```python
from build123d import *

# Parameters (mm, degrees)
SKETCH_1_R          = 1.6
EXTRUDE_1_DEPTH     = 13
SKETCH_2_W          = 16.5
SKETCH_2_H          = 11
CUT_EXTRUDE_1_DEPTH = 41.749969325
SKETCH_3_R          = 1.6
CUT_EXTRUDE_2_DEPTH = 34.189757456
FILLET_2_R          = 5
FILLET_3_R          = 3


with BuildPart() as part:
    # 草图1 → 凸台-拉伸1 (new, symmetric)
    with BuildSketch(Plane.XY):
        Polygon((-10.1, 0), (-10.1, 10), (10.1, 10), (10.1, 0), (13.1, 0), (26.6, 0), (26.6, 28), (10.6, 28), (10.6, 13), (-13.1, 13), (-13.1, 0), align=None)
        with Locations(Location((23.6, 25, 0), (0, 0, 180))):
            Circle(SKETCH_1_R, mode=Mode.SUBTRACT)
        with Locations(Location((13.6, 3, 0), (0, 0, 180))):
            Circle(SKETCH_1_R, mode=Mode.SUBTRACT)
    extrude(amount=EXTRUDE_1_DEPTH, both=True)

    # 草图2 → 切除-拉伸1 (cut, through all)
    with BuildSketch(Plane.XZ):
        with Locations((18.35, 0)):
            Rectangle(SKETCH_2_W, SKETCH_2_H)
    extrude(amount=-CUT_EXTRUDE_1_DEPTH, mode=Mode.SUBTRACT)

    # 草图3 → 切除-拉伸2 (cut, through all)
    with BuildSketch(Plane(origin=(0, 13, 0), x_dir=(1, 0, 0), z_dir=(0, 1, 0))):
        with Locations(Location((0, 10, 0), (0, 0, 180))):
            Circle(SKETCH_3_R)
        with Locations(Location((0, -10, 0), (0, 0, 180))):
            Circle(SKETCH_3_R)
    extrude(amount=-CUT_EXTRUDE_2_DEPTH, mode=Mode.SUBTRACT)

    # 圆角2
    fillet_2_edges = [part.edges().sort_by_distance(p)[0] for p in [
        (10.6, 13, -9.25),
    ]]
    fillet(fillet_2_edges, radius=FILLET_2_R)

    # 圆角3
    fillet_3_edges = [part.edges().sort_by_distance(p)[0] for p in [
        (10.6, 28, 9.25),
        (26.6, 28, 9.25),
        (26.6, 0, 9.25),
        (10.1, 0, 9.25),
        (10.6, 28, -9.25),
        (26.6, 28, -9.25),
        (26.6, 0, -9.25),
        (10.1, 0, -9.25),
    ]]
    fillet(fillet_3_edges, radius=FILLET_3_R)


solid = part.part
```
Build history of the part. All positions in model axes, mm. A direction names the side the tool comes from. Round coordinates to 2 decimals unless told otherwise and drop trailing zeros. Loops run counter-clockwise (first coordinate to the right, second up) from the corner with the lowest first, then second, coordinate; pieces in that order, holes last.
Item 1: Saw through at C-C (y = 10.75). List the corners of the cut face in (x, z), then the cut area to 3 significant figures.
Item 2: Pin check, flat tips, straight feed: P1, Ø3.5, axis at y = 22, z = -8.5, coming from the -X side; P2, Ø5, axis at x = 8.5, z = -10, coming from the +Y side; P3, Ø4, axis at x = 0, z = 10, coming from the +Y side. Stop position of each tip, or through.
Item 3: Drill centre lines: line 1 along X through (y, z) = (3, 8.5); line 2 along Y through (x, z) = (13.5, 11.5); line 3 along Y through (x, z) = (23.6, 7.5). Where is each one in solid material? Low to high.
Item 4: Saw through at A-A (z = -10). List the corners of the cut face in (x, y).
Item 5: Saw through at B-B (x = 0). List the corners of the cut face in (y, z), then the cut area to 3 significant figures.
Item 6: Saw through at D-D (x = 17). List the corners of the cut face in (y, z).
Item 7: Which spindle directions (+Z, -Z, +X, -X, +Y, -Y) get a long thin tool onto all of the face, cutting with end or side? Do faces 5 (the face through (10.6, 22, 9)), 6 (the face through (25.7, 27.14, -9.2)), 7 (the face through (0, 10, 0)). Say none if no direction does.
Item 8: Two-plate mould, pull along Y, no slides. Class faces 1 (the face through (11, 0.86, -9.2)), 2 (the face through (-4, 13, 0)), 3 (the face through (22, 25, 9)), 4 (the face through (26.6, 14, 9)): released by +Y, released by -Y, zero draft, split by the parting line, or undercut.
Worked answers:
1. outline: (-13.1, -13) - (26.6, -13) - (26.6, -5.5) - (10.1, -5.5) - (10.1, 5.5) - (26.6, 5.5) - (26.6, 13) - (-13.1, 13) - close; hole circle Ø3.2 at (0, -10); hole circle Ø3.2 at (0, 10)
1. area: 835 mm2
2. P1: stops at x = 10.6
2. P2: stops at y = 26.5
2. P3: stops at y = 13
3. line 1: x = -13.1 to -10.1, 10.1 to 12, 15.2 to 26.6
3. line 2: y = 0 to 1.4, 4.6 to 28
3. line 3: y = 0 to 23.4, 26.6 to 28
4. outline: (-13.1, 0) - (-10.1, 0) - (-10.1, 10) - (-1.6, 10) - (-1.6, 13) - (-13.1, 13) - close; (1.6, 10) - (10.1, 10) - (10.1, 3) arc R3 ccw to (13.1, 0) - (23.6, 0) arc R3 ccw to (26.6, 3) - (26.6, 25) arc R3 ccw to (23.6, 28) - (13.6, 28) arc R3 ccw to (10.6, 25) - (10.6, 18) arc R5 cw to (5.6, 13) - (1.6, 13) - close; hole circle Ø3.2 at (13.6, 3); hole circle Ø3.2 at (23.6, 25)
5. outline: (10, -13) - (13, -13) - (13, -11.6) - (10, -11.6) - close; (10, -8.4) - (13, -8.4) - (13, 8.4) - (10, 8.4) - close; (10, 11.6) - (13, 11.6) - (13, 13) - (10, 13) - close
5. area: 58.8 mm2
6. outline: (0, -13) - (28, -13) - (28, -5.5) - (0, -5.5) - close; (0, 5.5) - (28, 5.5) - (28, 13) - (0, 13) - close
7. face 5: +Z, -Z, -X, +Y
7. face 6: +Z, -Z, +X, +Y
7. face 7: +Z, -Z, -Y
8. face 1: released by -Y
8. face 2: released by +Y
8. face 3: undercut
8. face 4: zero draft
